The model under review builds one solid part; all positions refer to its coordinate system, in mm. A direction names the side the tool comes from. Round coordinates to 2 decimals unless told otherwise and drop trailing zeros. Loops run counter-clockwise (first coordinate to the right, second up) from the corner with the lowest first, then second, coordinate; pieces in that order, holes last. Notation, with made-up numbers: (-14.75, 15.25) -> (41.25, 15.25) arc R21 cw to (41.25, 25.25) -> close; hole circle Ø11 at (20.5, 78). An arc over 180 degrees is marked (long way). Use a Markdown table: item, result. Add a question column.
1) Mouldability with a two-part tool opening along X and no side actions: class faces 3 (the flat face through (249.56, 3, -42)), 4 (the flat face through (27.1, 3, -71)), 5 (the flat face through (0, 3, -42)), 6 (the flat face through (124, 0, -84)) as released by +X, released by -X, zero draft, split by the parting line, or undercut.
2) For faces 1 (the flat face through (24.1, 3, -71)), 2 (the flat face through (123, 3, 0)), list the 3-axis set-ups (+Z, -Z, +X, -X, +Y, -Y) from which the entire face can be reached by the end or side of a thin tool; tool diameter is ignored.
3) Consider section D-D on z = -8.5. Give the boundary of the cut face in (x, y), plus the area to 3 significant figures.
4) Insertion check: pin 1 (12 mm diameter, centred on x = 62.5, z = -11.5, fed in from -Y). The pin has a flat end and moves straight along its axis. Give the tip position at first contact, or say it passes through.
5) Consider section C-C on y = 4.05. Give the boundary of the cut face in (x, z).
6) Consider section A-A on x = 231.5. Give the boundary of the cut face in (y, z), plus the area to 3 significant figures.
7) Consider section B-B on z = -66. Give the boundary of the cut face in (x, y).
8) Wall thickness on probe 1 along X at (y, z) = (1.5, -71); probe 2 along Z at (x, y) = (223, 2.95); probe 3 along X at (y, z) = (5.05, -20): over which ranges is each line inside the solid? List them lowest first.
from build123d import *

# Parameters (mm, degrees)
ESQUISSE1_W        = 249.56
ESQUISSE1_H        = 85.25
BOSS_EXTRU_1_DEPTH = 6


with BuildPart() as part:
    # Esquisse1 → Boss.-Extru.1 (new body)
    with BuildSketch(Plane(origin=(0, 0, 0), x_dir=(1, 0, 0), z_dir=(0, 1, 0))):
        with Locations((124.78, 42.625)):
            Rectangle(ESQUISSE1_W, ESQUISSE1_H)
        Polygon((27.1, 81.25), (245.56, 81.25), (245.56, 4), (4, 4), (4, 81.25), (24.1, 81.25), (24.1, 61.15), (27.1, 61.15), align=None, mode=Mode.SUBTRACT)
    extrude(amount=BOSS_EXTRU_1_DEPTH)


solid = part.part
Result set:
| question | item | result |
|---|---|---|
| 1 | face 3 | released by +X |
| 1 | face 4 | undercut |
| 1 | face 5 | released by -X |
| 1 | face 6 | zero draft |
| 2 | face 1 | +Y, -Y |
| 2 | face 2 | +Z, +X, -X, +Y, -Y |
| 3 | outline | (0, 0) -> (4, 0) -> (4, 6) -> (0, 6) -> close; (245.56, 0) -> (249.56, 0) -> (249.56, 6) -> (245.56, 6) -> close |
| 3 | area | 48.0 mm2 |
| 4 | pin 1 | through |
| 5 | outline | (0, -85.25) -> (249.56, -85.25) -> (249.56, 0) -> (0, 0) -> close; hole (4, -81.25) -> (24.1, -81.25) -> (24.1, -61.15) -> (27.1, -61.15) -> (27.1, -81.25) -> (245.56, -81.25) -> (245.56, -4) -> (4, -4) -> close |
| 6 | outline | (0, -85.25) -> (6, -85.25) -> (6, -81.25) -> (0, -81.25) -> close; (0, -4) -> (6, -4) -> (6, 0) -> (0, 0) -> close |
| 6 | area | 48.0 mm2 |
| 7 | outline | (0, 0) -> (4, 0) -> (4, 6) -> (0, 6) -> close; (24.1, 0) -> (27.1, 0) -> (27.1, 6) -> (24.1, 6) -> close; (245.56, 0) -> (249.56, 0) -> (249.56, 6) -> (245.56, 6) -> close |
| 8 | probe 1 | 0 to 4, 24.1 to 27.1, 245.56 to 249.56 |
| 8 | probe 2 | -85.25 to -81.25, -4 to 0 |
| 8 | probe 3 | 0 to 4, 245.56 to 249.56 |
